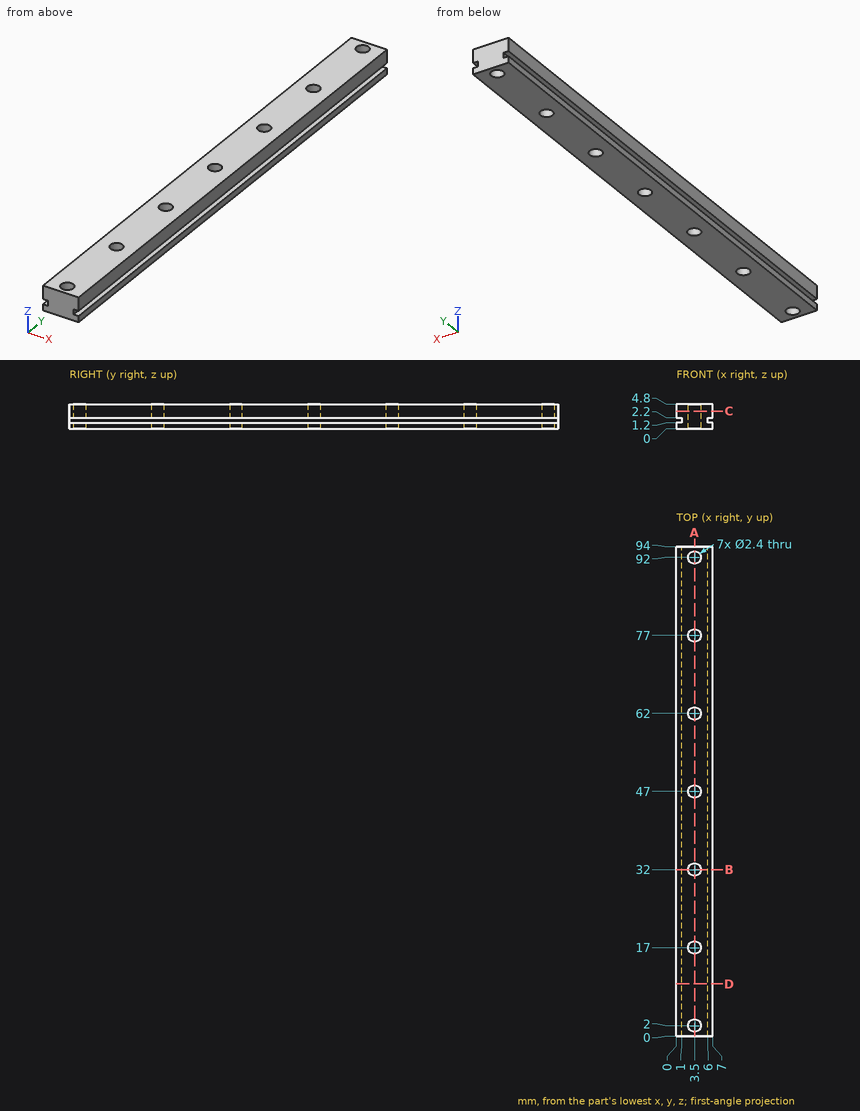
Design review of the part shown in the three views and the two pictorial views. Dimensions are in mm from the part's minimum x, y and z. Round coordinates to 2 decimals unless told otherwise and drop trailing zeros. Loops run counter-clockwise (first coordinate to the right, second up) from the corner with the lowest first, then second, coordinate; pieces in that order, holes last. Notation, with made-up numbers: (-26, 20.25) - (-2, 20.25) arc R11 cw to (-2, 30.25) - close; hole circle Ø2 at (12, -32.5). An arc over 180 degrees is marked (long way). Use CSV: the item, a comma, the result in double quotes.
(1) Take a section at B-B, the plane y = 32. Give the boundary of the cut face in (x, z).
Working result:
outline,"(0, 0) - (2.3, 0) - (2.3, 4.8) - (0, 4.8) - (0, 2.2) - (1, 2.2) - (1, 1.2) - (0, 1.2) - close; (4.7, 0) - (7, 0) - (7, 1.2) - (6, 1.2) - (6, 2.2) - (7, 2.2) - (7, 4.8) - (4.7, 4.8) - close"
(2) Clearance check with flat-ended pins moving along their axes: P1, Ø0.5, axis at y = 55.5, z = 2, coming from the +X side; P2, Ø1.9, axis at x = 3.5, y = 2, coming from the -Z side. State where each tip first meets the part, or that it passes through.
Working result:
P1,"stops at x = 7"
P2,"passes through"
(3) Take a section at D-D, the plane y = 10. Give the boundary of the cut face in (x, z).
Working result:
outline,"(0, 0) - (7, 0) - (7, 1.2) - (6, 1.2) - (6, 2.2) - (7, 2.2) - (7, 4.8) - (0, 4.8) - (0, 2.2) - (1, 2.2) - (1, 1.2) - (0, 1.2) - close"
(4) For line 1 (Z direction, x = 6.25, y = 68); line 2 (X direction, y = 77, z = 3.6); line 3 (X direction, y = 77.5, z = 3.3), list the stretches that pass through material, from the lowest coordinate up.
Working result:
line 1,"z = 0 to 1.2, 2.2 to 4.8"
line 2,"x = 0 to 2.3, 4.7 to 7"
line 3,"x = 0 to 2.41, 4.59 to 7"
(5) Take a section at C-C, the plane z = 3.45. Give the boundary of the cut face in (x, y), plus the area to 3 significant figures.
Working result:
outline,"(0, 0) - (7, 0) - (7, 94) - (0, 94) - close; hole circle Ø2.4 at (3.5, 2); hole circle Ø2.4 at (3.5, 17); hole circle Ø2.4 at (3.5, 32); hole circle Ø2.4 at (3.5, 47); hole circle Ø2.4 at (3.5, 62); hole circle Ø2.4 at (3.5, 77); hole circle Ø2.4 at (3.5, 92)"
area,"626 mm^2"
(6) Take a section at A-A, the plane x = 3.5. State how many separate pieces and enclosed holes the cut face has, plus the area to 3 significant figures.
Working result:
separate pieces,"8"
enclosed holes,"0"
area,"371 mm^2"
